```python
from build123d import *

# Parameters (mm, degrees)
SKETCH009_W     = 40.3725
SKETCH009_H     = 57.06
PAD005_DEPTH    = 1
SKETCH010_R     = 5.5
SKETCH010_R_2   = 4
SKETCH010_W     = 4.674176
SKETCH010_H     = 26.302142
POCKET003_DEPTH = 2
FILLET009_R     = 1
FILLET010_R     = 1
FILLET011_R     = 0.9
FILLET012_R     = 0.9
FILLET013_R     = 0.5


with BuildPart() as part:
    # Sketch009 → Pad005 (new body)
    with BuildSketch(Plane.XY.offset(10.9)):
        with Locations((16.18851, 26.244964)):
            Rectangle(SKETCH009_W, SKETCH009_H)
    extrude(amount=PAD005_DEPTH)

    # Sketch010 → Pocket003 (cut)
    with BuildSketch(Plane.XY.offset(11.9)):
        with Locations((23.106682, 26.030702)):
            Circle(SKETCH010_R)
        with Locations((23.106682, 12.530702)):
            Circle(SKETCH010_R_2)
        with Locations((6.364725, 18.636953)):
            Rectangle(SKETCH010_W, SKETCH010_H)
    extrude(amount=-POCKET003_DEPTH, mode=Mode.SUBTRACT)

    # Fillet009
    fillet009_edges = [part.edges().sort_by_distance(p)[0] for p in [
        (-3.99774, -2.285036, 11.4),
    ]]
    fillet(fillet009_edges, radius=FILLET009_R)

    # Fillet010
    fillet010_edges = [part.edges().sort_by_distance(p)[0] for p in [
        (36.37476, -2.285036, 11.4),
    ]]
    fillet(fillet010_edges, radius=FILLET010_R)

    # Fillet011
    fillet011_edges = [part.edges().sort_by_distance(p)[0] for p in [
        (36.37476, 54.774964, 11.4),
    ]]
    fillet(fillet011_edges, radius=FILLET011_R)

    # Fillet012
    fillet012_edges = [part.edges().sort_by_distance(p)[0] for p in [
        (-3.99774, 54.774964, 11.4),
    ]]
    fillet(fillet012_edges, radius=FILLET012_R)

    # Fillet013
    fillet013_edges = [part.edges().sort_by_distance(p)[0] for p in [
        (36.37476, 26.294964, 11.9),
    ]]
    fillet(fillet013_edges, radius=FILLET013_R)


solid = part.part
```
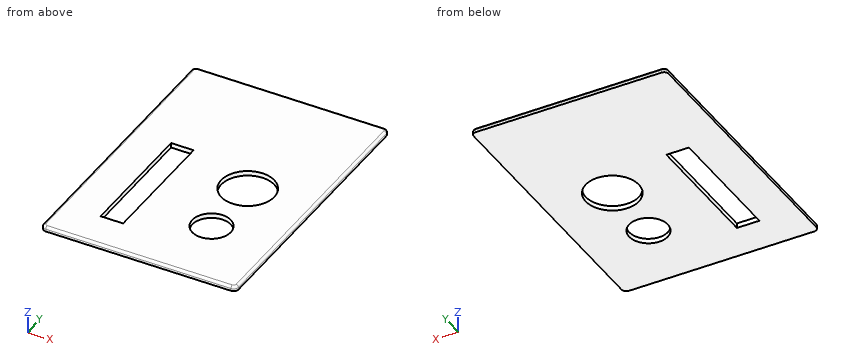
Build history of the part. All positions in model axes, mm. Give positions to 0.01 mm unless a question says otherwise; leave off trailing zeros. Loops run counter-clockwise (first coordinate to the right, second up) from the corner with the lowest first, then second, coordinate; pieces in that order, holes last. Notation, with made-up numbers: (59, 40.25) - (79, 40.25) arc R20 cw to (79, 78.25) - close; hole circle Ø3 at (-8.5, 9). An arc over 180 degrees is marked (long way). Use a Markdown table: item, result.
(1) Drop flat-ended pins along their axis: pin 1 Ø0.5 at (y, z) = (16.5, 11.5) entering from +X; pin 2 Ø7 at (x, y) = (23.11, 12.53) entering from +Z. Give the stop position or say it passes through.
Taken from the geometry:
| item | result |
|---|---|
| pin 1 | x = 36.37 |
| pin 2 | through |
(2) Wall check: line 1 along X through (y, z) = (29, 11.8); line 2 along X through (y, z) = (6.5, 11); line 3 along X through (y, z) = (11, 11.8). Give the ranges that are in metal, low to high.
Taken from the geometry:
| item | result |
|---|---|
| line 1 | -3.8 to 4.03, 8.7 to 18.48, 27.74 to 36.17 |
| line 2 | -4 to 4.03, 8.7 to 36.37 |
| line 3 | -3.8 to 4.03, 8.7 to 19.41, 26.8 to 36.17 |
(3) Band-saw the part on D-D (y = 28). Give the cut face in (x, z).
Taken from the geometry:
| item | result |
|---|---|
| outline | (-4, 10.9) - (4.03, 10.9) - (4.03, 11.9) - (-3.5, 11.9) arc R0.5 ccw to (-4, 11.4) - close; (8.7, 10.9) - (17.97, 10.9) - (17.97, 11.9) - (8.7, 11.9) - close; (28.24, 10.9) - (36.37, 10.9) - (36.37, 11.4) arc R0.5 ccw to (35.87, 11.9) - (28.24, 11.9) - close |
(4) Band-saw the part on B-B (y = 13.5). Give the cut face in (x, z), and give its area (3 significant figures).
Taken from the geometry:
| item | result |
|---|---|
| outline | (-4, 10.9) - (4.03, 10.9) - (4.03, 11.9) - (-3.5, 11.9) arc R0.5 ccw to (-4, 11.4) - close; (8.7, 10.9) - (19.23, 10.9) - (19.23, 11.9) - (8.7, 11.9) - close; (26.99, 10.9) - (36.37, 10.9) - (36.37, 11.4) arc R0.5 ccw to (35.87, 11.9) - (26.99, 11.9) - close |
| area | 27.8 mm2 |
(5) Band-saw the part on C-C (z = 11.2). Give the cut face in (x, y), and give its area (3 significant figures).
Taken from the geometry:
| item | result |
|---|---|
| outline | (-4, -1.29) arc R1 ccw to (-3, -2.29) - (35.37, -2.29) arc R1 ccw to (36.37, -1.29) - (36.37, 53.87) arc R0.9 ccw to (35.47, 54.77) - (-3.1, 54.77) arc R0.9 ccw to (-4, 53.87) - close; hole (4.03, 5.49) - (8.7, 5.49) - (8.7, 31.79) - (4.03, 31.79) - close; hole circle Ø11 at (23.11, 26.03); hole circle Ø8 at (23.11, 12.53) |
| area | 2,030 mm2 |
(6) Band-saw the part on A-A (x = 28). Give the cut face in (y, z).
Taken from the geometry:
| item | result |
|---|---|
| outline | (-2.29, 10.9) - (23.52, 10.9) - (23.52, 11.9) - (-1.79, 11.9) arc R0.5 ccw to (-2.29, 11.4) - close; (28.54, 10.9) - (54.77, 10.9) - (54.77, 11.4) arc R0.5 ccw to (54.27, 11.9) - (28.54, 11.9) - close |
